Build history of the part. All positions in model axes, mm. A direction names the side the tool comes from. Round coordinates to 2 decimals unless told otherwise and drop trailing zeros. Write each loop counter-clockwise with the first axis right and the second up, starting at its lowest first coordinate (ties: lowest second). Pieces come first, ordered by that corner, then holes.
Autodesk Inventor part; units mm, degrees
ref_plane "YZ Plane" through (0, 0, 0) normal (1, 0, 0) x (0, 1, 0)
ref_plane "XZ Plane" through (0, 0, 0) normal (0, 1, 0) x (-1, 0, 0)
ref_plane "XY Plane" through (0, 0, 0) normal (0, 0, 1) x (1, 0, 0)
sketch "Sketch1" plane through (0, 0, 0) normal (0, 1, 0) x (-1, 0, 0)
  line L0 (45, 22) -> (-45, 22)
  line L1 (-45, 22) -> (-45, -22)
  line L2 (-45, -22) -> (45, -22)
  line L3 (45, -22) -> (45, 22)
  line L4 (45, 22) -> (-45, -22) construction
  line L5 (-45, 22) -> (45, -22) construction
  point P0 (0, 0)
  dimension "d0" = 90
  dimension "d1" = 44
extrude "Extrusion1" add sketch "Sketch1" along normal blind 10
sketch "Sketch2" plane through (0, 10, 0) normal (0, 1, 0) x (1, 0, 0)
  line L0 (45, -22) -> (30, -22)
  line L1 (30, -22) -> (30, -17)
  line L2 (30, -17) -> (45, -17)
  line L3 (45, -17) -> (45, -22)
  line L4 (45, 17) -> (30, 17)
  line L5 (30, 17) -> (30, 22)
  line L6 (30, 22) -> (45, 22)
  line L7 (45, 22) -> (45, 17)
  line L8 (-45, -22) -> (-30, -22)
  line L9 (-30, -22) -> (-30, -17)
  line L10 (-30, -17) -> (-45, -17)
  line L11 (-45, -17) -> (-45, -22)
  line L12 (-45, 17) -> (-30, 17)
  line L13 (-30, 17) -> (-30, 22)
  line L14 (-30, 22) -> (-45, 22)
  line L15 (-45, 22) -> (-45, 17)
  line L16 (-45, 22) -> (-45, -22)
  line L17 (-45, -22) -> (45, -22)
  line L18 (45, 22) -> (-45, 22)
  line L19 (45, -22) -> (45, 22)
  point P0 (0, 0)
  dimension "d4" = 5
  dimension "d5" = 5
  dimension "d6" = 5
  dimension "d7" = 5
  dimension "d8" = 15
  dimension "d9" = 15
  dimension "d10" = 15
  dimension "d11" = 15
extrude "Extrusion2" add sketch "Sketch2" along normal blind 15 contours L0 L1 L2 L3 | L8 L11 L10 L9 | L4 L5 L6 L7 | L15 L14 L13 L12
sketch "Sketch3" plane through (-45, 0, 22) normal (0, 0, 1) x (1, 0, 0)
  circle A0 centre (82.5, 17.5) radius 2.05
  circle A1 centre (7.5, 17.5) radius 2.05
  line L0 (75, 25) -> (90, 25)
  line L1 (90, 0) -> (90, 25)
  line L2 (0, 25) -> (15, 25)
  line L3 (15, 10) -> (15, 25)
  point P0 (45, 0)
  point P1 (15, 17.5)
  dimension "d14" = 4.1
  dimension "d15" = 4.1
  dimension "d16" = 7.5
  dimension "d17" = 7.5
  dimension "d18" = 7.5
  dimension "d19" = 7.5
extrude "Extrusion3" cut sketch "Sketch3" against normal through all
sketch "Sketch6" plane through (0, 0, 0) normal (0, -1, 0) x (1, 0, 0)
  line L0 (-7.5, -7.5) -> (7.5, -7.5)
  line L1 (7.5, -7.5) -> (7.5, 7.5)
  line L2 (7.5, 7.5) -> (-7.5, 7.5)
  line L3 (-7.5, 7.5) -> (-7.5, -7.5)
  line L4 (-7.5, -7.5) -> (7.5, 7.5) construction
  line L5 (7.5, -7.5) -> (-7.5, 7.5) construction
  point P0 (0, 0)
  dimension "d27" = 15
  dimension "d28" = 15
extrude "Extrusion5" add sketch "Sketch6" along normal blind 15
sketch "Sketch7" plane through (7.5, 0, -7.5) normal (0, 0, -1) x (-1, 0, 0)
  circle A0 centre (7.5, -7.5) radius 4.5
  line L0 (-37.5, 0) -> (52.5, 0)
  line L1 (0, 0) -> (0, -15)
  point P0 (7.5, 0)
  dimension "d31" = 9
  dimension "d32" = 7.5
  dimension "d33" = 7.5
extrude "Extrusion6" cut sketch "Sketch7" against normal through all
sketch "Sketch8" plane through (-7.5, 0, 7.5) normal (0, 0, 1) x (1, 0, 0)
  line L0 (47.5, 0) -> (-32.5, 0)
  line L1 (-32.5, 0) -> (-32.5, -50)
  line L2 (-32.5, -50) -> (47.5, -50)
  line L3 (47.5, -50) -> (47.5, 0)
  line L4 (-37.5, 0) -> (52.5, 0)
  line L5 (0, 0) -> (0, -15)
  line L6 (15, -15) -> (0, -15)
  line L7 (15, 0) -> (15, -15)
  circle A0 centre (7.5, -7.5) radius 4.5
  line L8 (0, 0) -> (15, 0)
  line L9 (0, 0) -> (0, -15)
  line L10 (15, -15) -> (0, -15)
  line L11 (15, 0) -> (15, -15)
  point P0 (7.5, 0)
  point P1 (7.5, 0)
  dimension "d36" = 50
  dimension "d37" = 80
  dimension "d38" = 40
extrude "Extrusion7" add sketch "Sketch8" against normal blind 5 contours L3 L2 L1 L0 L5 L6 L7
sketch "Sketch10" plane through (-7.5, 0, 2.5) normal (0, 0, -1) x (-1, 0, 0)
  circle A0 centre (29.5, -47) radius 1.5
  circle A1 centre (-44.5, -47) radius 1.5
  circle A2 centre (29.5, -18) radius 1.5
  circle A3 centre (-44.5, -18) radius 1.5
  line L0 (-47.5, -50) -> (32.5, -50)
  line L1 (-47.5, 0) -> (-47.5, -50)
  line L2 (32.5, -50) -> (32.5, 0)
  point P0 (-7.5, 0)
  dimension "d58" = 3
  dimension "d59" = 3
  dimension "d60" = 3
  dimension "d61" = 3
  dimension "d62" = 3
  dimension "d63" = 3
  dimension "d64" = 3
  dimension "d65" = 3
  dimension "d66" = 29
  dimension "d67" = 29
  dimension "d68" = 3
  dimension "d69" = 3
extrude "Extrusion9" cut sketch "Sketch10" against normal blind 5
sketch "Sketch11" plane through (-7.5, 0, 2.5) normal (0, 0, -1) x (-1, 0, 0)
  circle A0 centre (-30.5, -40) radius 1.05
  circle A1 centre (15.5, -32.5) radius 1.05
  circle A2 centre (-30.5, -25) radius 1.05
  line L0 (-47.5, 0) -> (-47.5, -50)
  line L1 (-47.5, -50) -> (32.5, -50)
  point P0 (-7.5, 0)
  dimension "d75" = 2.1
  dimension "d76" = 2.1
  dimension "d77" = 2.1
  dimension "d78" = 46
  dimension "d79" = 7.5
  dimension "d80" = 7.5
  dimension "d81" = 17
  dimension "d82" = 0
  dimension "d83" = 10
extrude "Extrusion10" cut sketch "Sketch11" against normal through all
sketch "Sketch12" plane through (-7.5, 0, 2.5) normal (0, 0, -1) x (-1, 0, 0)
  line L0 (-3.5, -37.5) -> (-33.5, -37.5)
  line L1 (-33.5, -37.5) -> (-33.5, -27.5)
  line L2 (-33.5, -27.5) -> (-3.5, -27.5)
  line L3 (-3.5, -27.5) -> (-3.5, -37.5)
  line L4 (0, -15) -> (-15, -15)
  line L5 (-47.5, 0) -> (-47.5, -50)
  point P0 (-7.5, 0)
  dimension "d86" = 30
  dimension "d87" = 10
  dimension "d88" = 12.5
  dimension "d89" = 14
extrude "Extrusion11" cut sketch "Sketch12" against normal blind 10
sketch "Sketch13" plane through (-7.5, 0, 2.5) normal (0, 0, -1) x (-1, 0, 0)
  line L0 (18.5, -30.5) -> (6.5, -30.5)
  line L1 (6.5, -30.5) -> (6.5, -25.5)
  line L2 (6.5, -25.5) -> (18.5, -25.5)
  line L3 (18.5, -25.5) -> (18.5, -30.5)
  circle A0 centre (15.5, -32.5) radius 1.05
  line L4 (-3.5, -27.5) -> (-3.5, -37.5)
  point P0 (-7.5, 0)
  dimension "d92" = 5
  dimension "d93" = 2
  dimension "d94" = 3
  dimension "d97" = 12
extrude "Extrusion12" cut sketch "Sketch13" against normal through all contours L0 L1 L2 L3
properties part number "rail_top" material "ABS Plastic"
1) Mould opens along Y. For faces 5 (the flat face through (-45, 7, 0)), 6 (the flat face through (-1, -50, 5)), 7 (the cylindrical face through (-36.675, -48.464, 4.965)) say: released by +Y, released by -Y, zero draft, split by the parting line, or undercut.
Results:
face 5: zero draft
face 6: released by -Y
face 7: undercut
2) Slice it at D-D (y = -32.5). Write the cut outline in (x, z).
Results:
outline: (-40, 2.5) - (-24.05, 2.5) - (-24.05, 7.5) - (-40, 7.5) - close; (-21.95, 2.5) - (-4, 2.5) - (-4, 7.5) - (-21.95, 7.5) - close; (26, 2.5) - (40, 2.5) - (40, 7.5) - (26, 7.5) - close
3) Slice it at C-C (x = 23). Write the cut outline in (y, z), plus the area to 3 significant figures.
Results:
outline: (-50, 2.5) - (-41.05, 2.5) - (-41.05, 7.5) - (-50, 7.5) - close; (-38.95, 2.5) - (-37.5, 2.5) - (-37.5, 7.5) - (-38.95, 7.5) - close; (-27.5, 2.5) - (-26.05, 2.5) - (-26.05, 7.5) - (-27.5, 7.5) - close; (-23.95, 2.5) - (0, 2.5) - (0, -22) - (10, -22) - (10, 22) - (0, 22) - (0, 7.5) - (-23.95, 7.5) - close
area: 619 mm2
4) Pin check, flat tips, straight feed: pin 1 Ø1.5 at (x, y) = (34.5, -16.5) entering from -Z; pin 2 Ø5.5 at (x, z) = (13.5, 6) entering from +Y; pin 3 Ø3 at (x, y) = (20, -11) entering from +Z; pin 4 Ø1.9 at (x, y) = (-23, -32.5) entering from -Z. Stop position of each tip, or through.
Results:
pin 1: stops at z = 2.5
pin 2: stops at y = 10
pin 3: stops at z = 7.5
pin 4: passes through
5) Wall check: L1, parallel to Y at x = 37, z = 5.85; L2, parallel to X at y = 17, z = 20; L3, parallel to Y at x = 0, z = 2. Give the ranges that are in metal, low to high.
Results:
L1: y = -50 to -48.5, -45.5 to -19.5, -16.5 to 10
L2: x = -45 to -39.49, -35.51 to -30, 30 to 35.51, 39.49 to 45
L3: y = -15 to -12, -3 to 10
6) Slice it at A-A (x = -23). Write the cut outline in (y, z), plus the area to 4 significant figures.
Results:
outline: (-50, 2.5) - (-33.55, 2.5) - (-33.55, 7.5) - (-50, 7.5) - close; (-31.45, 2.5) - (-30.5, 2.5) - (-30.5, 7.5) - (-31.45, 7.5) - close; (-25.5, 2.5) - (0, 2.5) - (0, -22) - (10, -22) - (10, 22) - (0, 22) - (0, 7.5) - (-25.5, 7.5) - close
area: 654.5 mm2
7) Which spindle directions (+Z, -Z, +X, -X, +Y, -Y) get a long thin tool onto all of the face, cutting with end or side? Do faces 1 (the flat face through (30, 17, -19)), 2 (the flat face through (-26, -28, 5)), 3 (the flat face through (7.5, -7, -3)), 4 (the flat face through (-40, -25, 5)). Say none if no direction does.
Results:
face 1: +Z, -Z, +Y
face 2: +Z, -Z
face 3: -Z, +X, -Y
face 4: +Z, -Z, -X, -Y
8) Slice it at B-B (y = -7.5). Write the cut outline in (x, z), plus the area to 3 significant figures.
Results:
outline: (-40, 2.5) - (-7.5, 2.5) - (-7.5, -7.5) - (-4.5, -7.5) - (-4.5, 7.5) - (-40, 7.5) - close; (4.5, -7.5) - (7.5, -7.5) - (7.5, 2.5) - (40, 2.5) - (40, 7.5) - (4.5, 7.5) - close
area: 415 mm2
